from build123d import *

# Parameters (mm, degrees)
CROQUIS1_W              = 70
CROQUIS1_H              = 51.82
SALIENTE_EXTRUIR1_DEPTH = 72
CORTAR_EXTRUIR1_DEPTH   = 72
CROQUIS5_W              = 30
CROQUIS5_H              = 62
CORTAR_EXTRUIR2_DEPTH   = 35
CORTAR_EXTRUIR3_REACH   = 74
CROQUIS6_W              = 45
CROQUIS6_H              = 5
CORTAR_EXTRUIR4_REACH   = 53.82
CORTAR_EXTRUIR5_REACH   = 53.82
CROQUIS18_R             = 1.6
CORTAR_EXTRUIR7_DEPTH   = 15
CROQUIS19_R             = 1.75
CROQUIS19_R_2           = 2.5
CORTAR_EXTRUIR8_DEPTH   = 6
CORTAR_EXTRUIR10_DEPTH  = 10


with BuildPart() as part:
    # Croquis1 → Saliente-Extruir1 (new body)
    with BuildSketch(Plane(origin=(0, 0, 0), x_dir=(0, 0, -1), z_dir=(1, 0, 0))):
        with Locations((35, 25.91)):
            Rectangle(CROQUIS1_W, CROQUIS1_H)
    extrude(amount=SALIENTE_EXTRUIR1_DEPTH)

    # Croquis4 → Cortar-Extruir1 (cut)
    with BuildSketch(Plane(origin=(72, 0, 0), x_dir=(0, 0, -1), z_dir=(1, 0, 0))):
        Polygon((12.608406464, 30.515651581), (70, 0), (70, 51.82), (1.280683474, 51.82), align=None)
    extrude(amount=-CORTAR_EXTRUIR1_DEPTH, mode=Mode.SUBTRACT)

    # Croquis5 → Cortar-Extruir2 (cut)
    with BuildSketch(Plane(origin=(0, 51.82, 0), x_dir=(1, 0, 0), z_dir=(0, 1, 0))):
        with Locations((36, 31)):
            Rectangle(CROQUIS5_W, CROQUIS5_H)
    extrude(amount=-CORTAR_EXTRUIR2_DEPTH, mode=Mode.SUBTRACT)

    # Croquis6 → Cortar-Extruir3 (cut, up to next)
    with BuildSketch(Plane(origin=(72, 0, 0), x_dir=(0, 0, -1), z_dir=(1, 0, 0)), mode=Mode.PRIVATE) as cortar_extruir3_sk1:
        with Locations((22.5, 2.5)):
            Rectangle(CROQUIS6_W, CROQUIS6_H)
    cortar_extruir3_tool1 = extrude(cortar_extruir3_sk1.sketch, amount=-CORTAR_EXTRUIR3_REACH, mode=Mode.PRIVATE) & part.part
    add(cortar_extruir3_tool1.solids().sort_by_distance((72, 2.5, -22.5))[0], mode=Mode.SUBTRACT)

    # Croquis7 → Cortar-Extruir4 (cut, up to next)
    with BuildSketch(Plane(origin=(0, 51.82, 0), x_dir=(1, 0, 0), z_dir=(0, 1, 0)), mode=Mode.PRIVATE) as cortar_extruir4_sk1:
        Polygon((5.10343226, 0), (0, 1.280683474), (0, 0), align=None)
    cortar_extruir4_tool1 = extrude(cortar_extruir4_sk1.sketch, amount=-CORTAR_EXTRUIR4_REACH, mode=Mode.PRIVATE) & part.part
    add(cortar_extruir4_tool1.solids().sort_by_distance((1.701144, 51.82, -0.426894))[0], mode=Mode.SUBTRACT)

    # Croquis8 → Cortar-Extruir5 (cut, up to next)
    with BuildSketch(Plane(origin=(0, 51.82, 0), x_dir=(1, 0, 0), z_dir=(0, 1, 0)), mode=Mode.PRIVATE) as cortar_extruir5_sk1:
        Polygon((66.648328853, 0), (72, 10.382844773), (72, 0), align=None)
    cortar_extruir5_tool1 = extrude(cortar_extruir5_sk1.sketch, amount=-CORTAR_EXTRUIR5_REACH, mode=Mode.PRIVATE) & part.part
    add(cortar_extruir5_tool1.solids().sort_by_distance((70.21611, 51.82, -3.460948))[0], mode=Mode.SUBTRACT)

    # Croquis18 → Cortar-Extruir7 (cut)
    with BuildSketch(Plane.XY):
        with Locations((17.25, 23.32)):
            Circle(CROQUIS18_R)
        with Locations((54.25, 23.32)):
            Circle(CROQUIS18_R)
    extrude(amount=-CORTAR_EXTRUIR7_DEPTH, mode=Mode.SUBTRACT)

    # Croquis19 → Cortar-Extruir8 (cut)
    with BuildSketch(Plane.XZ.offset(-5)):
        with Locations((10, -35)):
            Circle(CROQUIS19_R)
        with Locations((10, -10)):
            Circle(CROQUIS19_R)
        with Locations((62, -35)):
            Circle(CROQUIS19_R)
        with Locations((62, -10)):
            Circle(CROQUIS19_R)
        with Locations((36, -35)):
            Circle(CROQUIS19_R_2)
        with Locations((36, -10)):
            Circle(CROQUIS19_R_2)
    extrude(amount=-CORTAR_EXTRUIR8_DEPTH, mode=Mode.SUBTRACT)

    # Croquis21 → Cortar-Extruir10 (cut)
    with BuildSketch(Plane.XY):
        Polygon((11.328328853, 5), (17.478328853, 5), (17.478328853, 17.92), (11.378328853, 17.92), align=None)
        Polygon((60.671671147, 5), (54.521671147, 5), (54.521671147, 17.92), (60.621671147, 17.92), align=None)
    extrude(amount=-CORTAR_EXTRUIR10_DEPTH, mode=Mode.SUBTRACT)


solid = part.part
Could you check a few things on this model? Use its own coordinates, in mm. A direction names the side the tool comes from. Round coordinates to 2 decimals unless told otherwise and drop trailing zeros. Order: outer loops, then holes, each group sorted by start corner. A loop starts at its lowest first (then second) coordinate and runs counter-clockwise, first axis right, second up.
(1) Imagine slicing it at D-D (y = 36.5). Write out the boundary of the cut face in (x, z), plus the area to 3 significant figures.
Response values:
outline: (0, -9.43) - (21, -9.43) - (21, 0) - (5.1, 0) - (0, -1.28) - close; (51, -9.43) - (71.51, -9.43) - (66.65, 0) - (51, 0) - close
area: 365 mm2
(2) Which directions (+Z, -Z, +X, -X, +Y, -Y) give clear straight access to the entire face, cutting with the end or side of a thin tool? Please do faces 5 (the flat face through (17, 23, -15)), 6 (the flat face through (58, 12, -10)), 7 (the flat face through (35, 0, -57)), 8 (the cylindrical face through (38.385, 7.958, -34.249)), 9 (the flat face through (37, 2, -45)).
Response values:
face 5: +Z
face 6: +Z, -Y
face 7: +Z, -Z, +X, -X, -Y
face 8: -Y
face 9: +Z, +X, -X, -Y
(3) Please list where these lines run through material, in increasing order: line 1 along Z through (x, y) = (36, 6); line 2 along Z through (x, y) = (62, 8); line 3 along Y through (x, z) = (43.5, -26.5).
Response values:
line 1: z = -58.72 to -37.5, -32.5 to -12.5, -7.5 to 0
line 2: z = -54.95 to -36.75, -33.25 to -11.75, -8.25 to 0
line 3: y = 5 to 16.82
(4) Imagine slicing it at C-C (z = -18). Write out the boundary of the cut face in (x, y).
Response values:
outline: (0, 5) - (72, 5) - (72, 27.65) - (51, 27.65) - (51, 16.82) - (21, 16.82) - (21, 27.65) - (0, 27.65) - close
(5) If we mould it in two halves opening along Z, with no side actions, what happens to faces 1 (the flat face through (2.59, 28.74, -0.63)), 2 (the flat face through (17.478, 11, -5)), 3 (the flat face through (62, 11, -10)), 4 (the cylindrical face through (63.617, 7.958, -35.67))? For each: released by +Z, released by -Z, zero draft, split by the parting line, or undercut.
Response values:
face 1: released by +Z
face 2: zero draft
face 3: undercut
face 4: undercut
(6) Imagine slicing it at A-A (y = 23.32). Write out the boundary of the cut face in (x, z).
Response values:
outline: (0, -26.14) - (21, -26.14) - (21, 0) - (18.85, 0) - (18.85, -15) - (15.65, -15) - (15.65, 0) - (5.1, 0) - (0, -1.28) - close; (51, -26.14) - (72, -26.14) - (72, -10.38) - (66.65, 0) - (55.85, 0) - (55.85, -15) - (52.65, -15) - (52.65, 0) - (51, 0) - close
(7) I'm going to push flat-ended pins straight in: pin 1 (1.5 mm diameter, centred on x = 35.5, z = -36, fed in from -Y); pin 2 (2 mm diameter, centred on x = 11.5, y = 33, fed in from -Z); pin 3 (5 mm diameter, centred on x = 14.5, z = -3, fed in from -Y). Where does each tip first touch, or does it pass through?
Response values:
pin 1: stops at y = 11
pin 2: stops at z = -11.82
pin 3: stops at y = 17.92
(8) Imagine slicing it at B-B (x = 36). Write out the boundary of the cut face in (y, z).
Response values:
outline: (0, -70) - (16.82, -38.37) - (16.82, 0) - (5, 0) - (5, -7.5) - (11, -7.5) - (11, -12.5) - (5, -12.5) - (5, -32.5) - (11, -32.5) - (11, -37.5) - (5, -37.5) - (5, -45) - (0, -45) - close
